Source: three-view drawing plus pictorial views. Frame: mm from the lowest corner of the part. A direction names the side the tool comes from. Coordinates: 2 decimals unless noted, no trailing zeros. Write each loop counter-clockwise with the first axis right and the second up, starting at its lowest first coordinate (ties: lowest second). Pieces come first, ordered by that corner, then holes. Notation, with made-up numbers: M 65,66.25 L 101,66.25 A32 cw 101,100.25 Z; hole C -35.5,49 d4. An arc over 180 degrees is marked long. Write item = value, one per line. Start each with the question number.
Item 1: Section A-A on y = 3.7. Output: boundary loops of the cut face in (x, z).
Item 2: Ray query, L1, parallel to Y at x = 12.2, z = 52.8; L2, parallel to Y at x = 12.2, z = 54.55; L3, parallel to Z at x = 15.75, y = 8. Return the intervals inside material, ascending. Write a range as [from, to].
Item 3: First-contact query: pin 1 Ø1.5 at (x, z) = (9.5, 40.5) entering from +Y; pin 2 Ø12 at (y, z) = (18.5, 12) entering from -X; pin 3 Ø1 at (x, z) = (8.5, 11.5) entering from -Y. Flat tips, straight axial feed; report the tip coordinate or a pass-through.
Item 4: Reachability of the marked faces 1 and 2 from +Z, -Z, +X, -X, +Y, -Y: full face, straight path, thin tool, end or side. Return the list, or none.
Item 5: Section D-D on x = 19.5. Output: boundary loops of the cut face in (y, z), plus the area to 3 significant figures.
Item 6: Section C-C on z = 11.5. Output: boundary loops of the cut face in (x, y), plus the area to 3 significant figures.
Item 7: Section B-B on x = 12.2. Output: boundary loops of the cut face in (y, z).
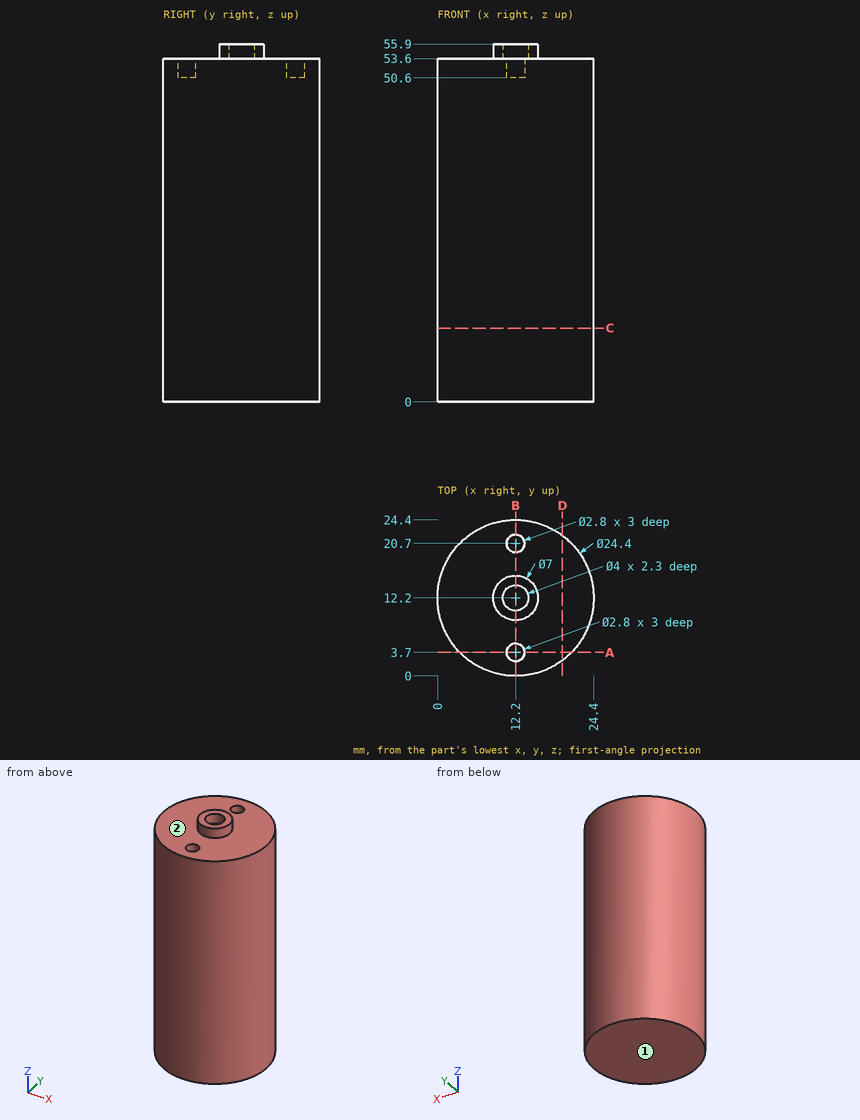
Responses:
q1.outline = M 3.45,0 L 20.95,0 L 20.95,53.6 L 13.6,53.6 L 13.6,50.6 L 10.8,50.6 L 10.8,53.6 L 3.45,53.6 Z
q2.L1 = [0, 2.3], [5.1, 19.3], [22.1, 24.4]
q2.L2 = [8.7, 10.2], [14.2, 15.7]
q2.L3 = [0, 53.6]
q3.pin_1 = 24.24
q3.pin_2 = 0
q3.pin_3 = 0.43
q4.face_1 = -Z, +X, -X, +Y, -Y
q4.face_2 = +Z
q5.outline = M 2.43,0 L 21.97,0 L 21.97,53.6 L 2.43,53.6 Z
q5.area = 1,050 mm²
q6.outline = C 12.2,12.2 d24.4
q6.area = 468 mm²
q7.outline = M 0,0 L 24.4,0 L 24.4,53.6 L 22.1,53.6 L 22.1,50.6 L 19.3,50.6 L 19.3,53.6 L 15.7,53.6 L 15.7,55.9 L 14.2,55.9 L 14.2,53.6 L 10.2,53.6 L 10.2,55.9 L 8.7,55.9 L 8.7,53.6 L 5.1,53.6 L 5.1,50.6 L 2.3,50.6 L 2.3,53.6 L 0,53.6 Z
